from build123d import *

# Parameters (mm, degrees)
BOSS_EXTRU_1_DEPTH      = 10
ENL_V_MAT_EXTRU_1_REACH = 128.984
ESQUISSE2_R             = 1.75
ESQUISSE4_R             = 3.5
ENL_V_MAT_EXTRU_2_DEPTH = 4
ESQUISSE5_W             = 50
ESQUISSE5_H             = 38
BOSS_EXTRU_2_DEPTH      = 14.4
ENL_V_MAT_EXTRU_3_REACH = 56.766
ESQUISSE6_R             = 1.5
ESQUISSE7_R             = 3
ENL_V_MAT_EXTRU_4_DEPTH = 9.4
CHANFREIN1_SIZE         = 10
CHANFREIN2_SIZE         = 28
CHANFREIN2_SIZE_2       = 10
BOSS_EXTRU_3_DEPTH      = 5
ESQUISSE9_W             = 38
ESQUISSE9_H             = 28.6
BOSS_EXTRU_4_DEPTH      = 2.5
CHANFREIN3_SIZE         = 5
ENL_V_MAT_EXTRU_5_REACH = 143.753
ESQUISSE10_R            = 1.5
ESQUISSE11_R            = 3
ENL_V_MAT_EXTRU_6_DEPTH = 2.5


# Some blends are built 0.0001 mm under size
with BuildPart() as part:
    # Esquisse1 → Boss.-Extru.1 (new body)
    with BuildSketch(Plane.XY):
        with BuildLine():
            Line((-20, -123.389626793), (-20, -99.4))
            Line((-20, -99.4), (20, -99.4))
            Line((20, -99.4), (20, -123.389626793))
            ThreePointArc((20, -123.389626793), (0, -125), (-20, -123.389626793))
        make_face()
    extrude(amount=BOSS_EXTRU_1_DEPTH)

    # Esquisse2 → Enlèv. mat.-Extru.1 (cut, up to next)
    with BuildSketch(Plane.XY.offset(10), mode=Mode.PRIVATE) as enl_v_mat_extru_1_sk1:
        with Locations((-10, -110)):
            Circle(ESQUISSE2_R)
    enl_v_mat_extru_1_tool1 = extrude(enl_v_mat_extru_1_sk1.sketch, amount=-ENL_V_MAT_EXTRU_1_REACH, mode=Mode.PRIVATE) & part.part
    # Esquisse2 → Enlèv. mat.-Extru.1 (cut, up to next)
    with BuildSketch(Plane.XY.offset(10), mode=Mode.PRIVATE) as enl_v_mat_extru_1_sk2:
        with Locations((-10, -120)):
            Circle(ESQUISSE2_R)
    enl_v_mat_extru_1_tool2 = extrude(enl_v_mat_extru_1_sk2.sketch, amount=-ENL_V_MAT_EXTRU_1_REACH, mode=Mode.PRIVATE) & part.part
    # Esquisse2 → Enlèv. mat.-Extru.1 (cut, up to next)
    with BuildSketch(Plane.XY.offset(10), mode=Mode.PRIVATE) as enl_v_mat_extru_1_sk3:
        with Locations((10, -110)):
            Circle(ESQUISSE2_R)
    enl_v_mat_extru_1_tool3 = extrude(enl_v_mat_extru_1_sk3.sketch, amount=-ENL_V_MAT_EXTRU_1_REACH, mode=Mode.PRIVATE) & part.part
    # Esquisse2 → Enlèv. mat.-Extru.1 (cut, up to next)
    with BuildSketch(Plane.XY.offset(10), mode=Mode.PRIVATE) as enl_v_mat_extru_1_sk4:
        with Locations((10, -120)):
            Circle(ESQUISSE2_R)
    enl_v_mat_extru_1_tool4 = extrude(enl_v_mat_extru_1_sk4.sketch, amount=-ENL_V_MAT_EXTRU_1_REACH, mode=Mode.PRIVATE) & part.part
    add(enl_v_mat_extru_1_tool1.solids().sort_by_distance((-10, -110, 10))[0], mode=Mode.SUBTRACT)
    add(enl_v_mat_extru_1_tool2.solids().sort_by_distance((-10, -120, 10))[0], mode=Mode.SUBTRACT)
    add(enl_v_mat_extru_1_tool3.solids().sort_by_distance((10, -110, 10))[0], mode=Mode.SUBTRACT)
    add(enl_v_mat_extru_1_tool4.solids().sort_by_distance((10, -120, 10))[0], mode=Mode.SUBTRACT)

    # Esquisse4 → Enlèv. mat.-Extru.2 (cut)
    with BuildSketch(Plane.XY.offset(10)):
        with Locations((-10, -110)):
            Circle(ESQUISSE4_R)
        with Locations((10, -110)):
            Circle(ESQUISSE4_R)
        with Locations((10, -120)):
            Circle(ESQUISSE4_R)
        with Locations((-10, -120)):
            Circle(ESQUISSE4_R)
    extrude(amount=-ENL_V_MAT_EXTRU_2_DEPTH, mode=Mode.SUBTRACT)

    # Esquisse5 → Boss.-Extru.2 (add)
    with BuildSketch(Plane(origin=(0, -99.4, 0), x_dir=(1, 0, 0), z_dir=(0, 1, 0))):
        with Locations((5, -19)):
            Rectangle(ESQUISSE5_W, ESQUISSE5_H)
    extrude(amount=BOSS_EXTRU_2_DEPTH)

    # Esquisse6 → Enlèv. mat.-Extru.3 (cut, up to next)
    with BuildSketch(Plane.XZ.offset(99.4), mode=Mode.PRIVATE) as enl_v_mat_extru_3_sk1:
        with Locations(Location((-2, 27, 0), (0, 0, 270))):
            Circle(ESQUISSE6_R)
    enl_v_mat_extru_3_tool1 = extrude(enl_v_mat_extru_3_sk1.sketch, amount=-ENL_V_MAT_EXTRU_3_REACH, mode=Mode.PRIVATE) & part.part
    # Esquisse6 → Enlèv. mat.-Extru.3 (cut, up to next)
    with BuildSketch(Plane.XZ.offset(99.4), mode=Mode.PRIVATE) as enl_v_mat_extru_3_sk2:
        with Locations(Location((22, 27, 0), (0, 0, 270))):
            Circle(ESQUISSE6_R)
    enl_v_mat_extru_3_tool2 = extrude(enl_v_mat_extru_3_sk2.sketch, amount=-ENL_V_MAT_EXTRU_3_REACH, mode=Mode.PRIVATE) & part.part
    # Esquisse6 → Enlèv. mat.-Extru.3 (cut, up to next)
    with BuildSketch(Plane.XZ.offset(99.4), mode=Mode.PRIVATE) as enl_v_mat_extru_3_sk3:
        with Locations(Location((-2, 15, 0), (0, 0, 270))):
            Circle(ESQUISSE6_R)
    enl_v_mat_extru_3_tool3 = extrude(enl_v_mat_extru_3_sk3.sketch, amount=-ENL_V_MAT_EXTRU_3_REACH, mode=Mode.PRIVATE) & part.part
    # Esquisse6 → Enlèv. mat.-Extru.3 (cut, up to next)
    with BuildSketch(Plane.XZ.offset(99.4), mode=Mode.PRIVATE) as enl_v_mat_extru_3_sk4:
        with Locations(Location((22, 15, 0), (0, 0, 270))):
            Circle(ESQUISSE6_R)
    enl_v_mat_extru_3_tool4 = extrude(enl_v_mat_extru_3_sk4.sketch, amount=-ENL_V_MAT_EXTRU_3_REACH, mode=Mode.PRIVATE) & part.part
    add(enl_v_mat_extru_3_tool1.solids().sort_by_distance((-2, -99.4, 27))[0], mode=Mode.SUBTRACT)
    add(enl_v_mat_extru_3_tool2.solids().sort_by_distance((22, -99.4, 27))[0], mode=Mode.SUBTRACT)
    add(enl_v_mat_extru_3_tool3.solids().sort_by_distance((-2, -99.4, 15))[0], mode=Mode.SUBTRACT)
    add(enl_v_mat_extru_3_tool4.solids().sort_by_distance((22, -99.4, 15))[0], mode=Mode.SUBTRACT)

    # Esquisse7 → Enlèv. mat.-Extru.4 (cut)
    with BuildSketch(Plane.XZ.offset(99.4)):
        with Locations(Location((-2, 27, 0), (0, 0, 270))):
            Circle(ESQUISSE7_R)
        with Locations(Location((22, 27, 0), (0, 0, 270))):
            Circle(ESQUISSE7_R)
        with Locations(Location((22, 15, 0), (0, 0, 270))):
            Circle(ESQUISSE7_R)
        with Locations(Location((-2, 15, 0), (0, 0, 270))):
            Circle(ESQUISSE7_R)
    extrude(amount=-ENL_V_MAT_EXTRU_4_DEPTH, mode=Mode.SUBTRACT)

    # Chanfrein1
    chanfrein1_edges = [part.edges().sort_by_distance(p)[0] for p in [
        (30, -92.2, 0),
    ]]
    chamfer(chanfrein1_edges, length=CHANFREIN1_SIZE)

    # Chanfrein2
    # the kernel refuses this chamfer: 28, 10 mm, written as the material it takes off along each edge
    with BuildSketch(Plane(origin=(102.642981969, -99.4, 38), x_dir=(0, -0.01296397650632004, -0.9999159641255577), z_dir=(-1, 0, 0))) as chanfrein2_piece_1:
        Polygon((CHANFREIN2_SIZE * 0.999915964126, -CHANFREIN2_SIZE * 0.0129639765063), (-CHANFREIN2_SIZE_2 * 0.0129639765063, -CHANFREIN2_SIZE_2 * 0.999915964126), (0, 0), align=None)
    extrude(amount=195.285963938, mode=Mode.SUBTRACT)

    # Esquisse8 → Boss.-Extru.3 (add)
    with BuildSketch(Plane.ZY.offset(20)):
        Polygon((10, -99.4), (0, -99.4), (0, -56.4), (38, -56.4), (38, -89.4), align=None)
    extrude(amount=BOSS_EXTRU_3_DEPTH)

    # Esquisse9 → Boss.-Extru.4 (add)
    with BuildSketch(Plane(origin=(-20, 0, 0), x_dir=(0, 0, -1), z_dir=(1, 0, 0))):
        with Locations((-19, -70.7)):
            Rectangle(ESQUISSE9_W, ESQUISSE9_H)
    extrude(amount=BOSS_EXTRU_4_DEPTH)

    # Chanfrein3
    chanfrein3_edges = [part.edges().sort_by_distance(p)[0] for p in [
        (-20, -99.4, 5),
    ]]
    chamfer(chanfrein3_edges, length=CHANFREIN3_SIZE - 0.0001)  # a hair under: the kernel refuses the full size

    # Esquisse10 → Enlèv. mat.-Extru.5 (cut, up to next)
    with BuildSketch(Plane.ZY.offset(25), mode=Mode.PRIVATE) as enl_v_mat_extru_5_sk1:
        with Locations(Location((15, -62.75, 0), (0, 0, 270))):
            Circle(ESQUISSE10_R)
    enl_v_mat_extru_5_tool1 = extrude(enl_v_mat_extru_5_sk1.sketch, amount=-ENL_V_MAT_EXTRU_5_REACH, mode=Mode.PRIVATE) & part.part
    # Esquisse10 → Enlèv. mat.-Extru.5 (cut, up to next)
    with BuildSketch(Plane.ZY.offset(25), mode=Mode.PRIVATE) as enl_v_mat_extru_5_sk2:
        with Locations(Location((15, -78.75, 0), (0, 0, 270))):
            Circle(ESQUISSE10_R)
    enl_v_mat_extru_5_tool2 = extrude(enl_v_mat_extru_5_sk2.sketch, amount=-ENL_V_MAT_EXTRU_5_REACH, mode=Mode.PRIVATE) & part.part
    add(enl_v_mat_extru_5_tool1.solids().sort_by_distance((-25, -62.75, 15))[0], mode=Mode.SUBTRACT)
    add(enl_v_mat_extru_5_tool2.solids().sort_by_distance((-25, -78.75, 15))[0], mode=Mode.SUBTRACT)

    # Esquisse11 → Enlèv. mat.-Extru.6 (cut)
    with BuildSketch(Plane.ZY.offset(25)):
        with Locations(Location((15, -62.75, 0), (0, 0, 270))):
            Circle(ESQUISSE11_R)
        with Locations(Location((15, -78.75, 0), (0, 0, 270))):
            Circle(ESQUISSE11_R)
    extrude(amount=-ENL_V_MAT_EXTRU_6_DEPTH, mode=Mode.SUBTRACT)


solid = part.part
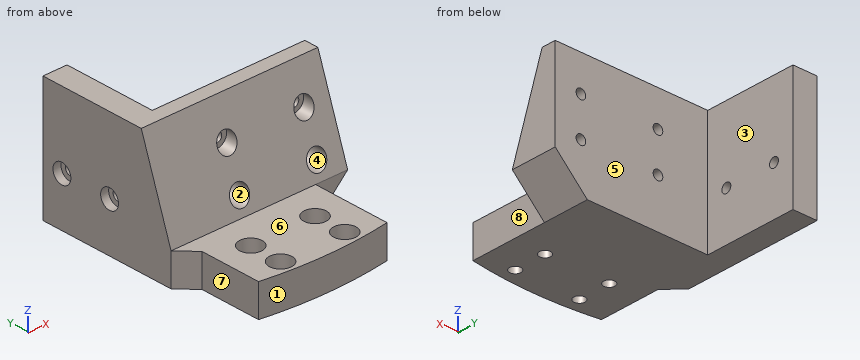
Model file for the job. Use its own axes, mm. Face numbers are marked on the shaded views. A direction names the side the tool comes from. Give positions to 0.01 mm unless a question says otherwise; leave off trailing zeros. Order: outer loops, then holes, each group sorted by start corner. A loop starts at its lowest first (then second) coordinate and runs counter-clockwise, first axis right, second up. Notation, with made-up numbers: M -8.5,-40 L 49.5,-40 A17 cw 49.5,-20 Z; hole C 15.25,31 d8. An arc over 180 degrees is marked long. Put each result on its own line as item: value. Start each with the question number.
(1) Band-saw the part on C-C on x = 22. Give the cut face in (y, z), then the cut area to 3 significant figures.
(2) Band-saw the part on B-B on y = -110. Give the cut face in (x, z), then the cut area to 3 significant figures.
(3) Pull direction X, two halves, no side cores. Call the marked faces 1, 2, 3 and 4: released by +X, released by -X, zero draft, split by the parting line, or undercut.
(4) Pin check, flat tips, straight feed: pin 1 Ø1.5 at (x, z) = (21, 28) entering from -Y; pin 2 Ø8 at (x, z) = (14, 5.5) entering from +Y; pin 3 Ø3.5 at (x, y) = (-11.5, -108.5) entering from +Z; pin 4 Ø3 at (x, y) = (10, -120) entering from +Z. Stop position of each tip, or through.
(5) Band-saw the part on A-A on y = -78.75. Give the cut face in (x, z).
(6) Band-saw the part on D-D on z = 34.5. Give the cut face in (x, y), then the cut area to 3 significant figures.
(7) Drill centre lines: L1, parallel to X at y = -91.1, z = 27; L2, parallel to Y at x = 10, z = 7; L3, parallel to X at y = -120, z = 1.8. Where is each one in solid material? Low to high. Write a range as [from, to].
(8) Tool access for the marked faces 5, 6, 7 and 8: list every direction of +Z, -Z, +X, -X, +Y, -Y with a clear straight run to the whole face (end or side of a thin tool).
Results below:
1. outline: M -99.4,2 L -85,2 L -85,13.5 L -90,13.5 L -90,12 L -98.69,12 L -99.4,10 Z; M -96.54,18 L -90,18 L -90,16.5 L -85,16.5 L -85,25.5 L -90,25.5 L -90,24 L -94.4,24 Z; M -92.26,30 L -90,30 L -90,28.5 L -85,28.5 L -85,38 L -89.4,38 Z
1. area: 283 mm2
2. outline: M -20,0 L -11.75,0 L -11.75,6 L -13.5,6 L -13.5,10 L -20,10 Z; M -8.25,0 L 8.25,0 L 8.25,6 L 6.5,6 L 6.5,10 L -6.5,10 L -6.5,6 L -8.25,6 Z; M 11.75,0 L 20,0 L 20,10 L 13.5,10 L 13.5,6 L 11.75,6 Z
2. area: 302 mm2
3. face 1: split by the parting line
3. face 2: undercut
3. face 3: released by +X
3. face 4: undercut
4. pin 1: stops at y = -90
4. pin 2: stops at y = -85
4. pin 3: stops at z = 10
4. pin 4: passes through
5. outline: M -25,0 L -17.5,0 L -17.5,13.5 L -22.5,13.5 L -22.5,12 L -25,12 Z; M -25,18 L -22.5,18 L -22.5,16.5 L -17.5,16.5 L -17.5,38 L -25,38 Z
6. outline: M -25,-90.65 L 30,-90.65 L 30,-85 L -17.5,-85 L -17.5,-56.4 L -25,-56.4 Z
6. area: 525 mm2
7. L1: x = [-25, -5], [1, 19], [25, 30]
7. L2: y = [-124.6, -123.5], [-116.5, -113.5], [-106.5, -85]
7. L3: x = [-20, -11.75], [-8.25, 8.25], [11.75, 20]
8. face 5: +Z, -Z, +X, +Y
8. face 6: +Z, +X, -X, -Y
8. face 7: +Z, -Z, -X, -Y
8. face 8: +Z, -Z, +X, -Y
